Verification items for the finished model (mm, model axes). Coordinates: 2 decimals unless noted, no trailing zeros. Order: outer loops, then holes, each group sorted by start corner. A loop starts at its lowest first (then second) coordinate and runs counter-clockwise, first axis right, second up. Notation, with made-up numbers: M 78.25,62 L 90.25,62 A27 ccw 90.25,80 Z; hole C -6.75,84.25 d1. An arc over 180 degrees is marked long. Return JSON: item names as keys, results as strings. Group by question number.
Q1. Thickness scan on probe 1 along Y at (x, z) = (126.16, 2.05); probe 2 along Y at (x, z) = (33, 0.2); probe 3 along Y at (x, z) = (14, 2.6). Record the ranges inside material, lowest first.
Q2. Section check A-A, the plane z = 1.95. Count the separate pieces of the cut face and the enclosed holes in it, then the cut area to 3 significant figures.
Q3. Go/stop test with flat-tipped pins: pin 1 Ø0.6 at (y, z) = (190, 2) entering from -X; pin 2 Ø1 at (x, z) = (42.5, 1.5) entering from +Y. Record where each tip stops, or that it passes through.
Q4. Mould release check, pull along X, two halves, no side actions. Record for faces 1 (the face through (120.064, 179.912, 1.521)), 2 (the face through (91.605, 168.618, 1.479)), 3 (the face through (93, 63, 3)): pulls with the +X half, pulls with the -X half, needs draft (parallel to the pull), parting line crosses it, or undercut.
Q5. Section check C-C, the plane x = 56.5. Enter the section's corners in (y, z), then the cut area to 3 significant figures.
Q6. Section check B-B, the plane y = -30. Enter the section's corners in (x, z), then the cut area to 3 significant figures.
Autodesk Inventor part; units mm, degrees
ref_plane "YZ Plane" through (0, 0, 0) normal (1, 0, 0) x (0, 1, 0)
ref_plane "XZ Plane" through (0, 0, 0) normal (0, 1, 0) x (-1, 0, 0)
ref_plane "XY Plane" through (0, 0, 0) normal (0, 0, 1) x (1, 0, 0)
sketch "スケッチ1" plane through (0, 0, 0) normal (0, 0, 1) x (1, 0, 0)
  line L0 (0, 0) -> (130.16, 0)
  line L1 (130.16, 0) -> (130.16, 159.597)
  line L2 (130.16, 159.597) -> (0, 159.597)
  line L3 (0, 159.597) -> (0, 0)
  dimension "d0" = 130.16
  dimension "d1" = 159.597
extrude "押し出し1" add sketch "スケッチ1" along normal blind 3
sketch "スケッチ2" plane through (0, 0, 3) normal (0, 0, 1) x (1, 0, 0)
  line L0 (126.16, 3.92) -> (126.16, 113.08) construction
  circle A0 centre (126.16, 3.92) radius 1.6
  circle A1 centre (126.16, 113.08) radius 1.6
  line L1 (130.16, 0) -> (130.16, 159.597)
  line L2 (0, 0) -> (130.16, 0)
  circle A2 centre (121.531, 154.597) radius 1.6
  line L3 (130.16, 159.597) -> (0, 159.597)
  line L4 (121.531, 154.597) -> (121.531, 139.097) construction
  circle A3 centre (121.531, 139.097) radius 1.6
  line L5 (18.398, 154.597) -> (33.898, 154.597) construction
  line L6 (0, 159.597) -> (0, 0) construction
  circle A4 centre (18.398, 154.597) radius 1.6
  circle A5 centre (33.898, 154.597) radius 1.6
  dimension "d4" = 3.2
  dimension "d5" = 4
  dimension "d6" = 3.92
  dimension "d7" = 109.16
  dimension "d10" = 5
  dimension "d11" = 8.629
  dimension "d12" = 15.5
  dimension "d13" = 18.398
  dimension "d14" = 5
  dimension "d15" = 15.5
extrude "押し出し2" cut sketch "スケッチ2" against normal blind 3
sketch "スケッチ9" plane through (0, 0, 3) normal (0, 0, 1) x (1, 0, 0)
  line L0 (130.16, 159.597) -> (0, 159.597)
  line L1 (100.16, 192.597) -> (130.16, 192.597)
  line L2 (130.16, 192.597) -> (130.16, 159.597)
  line L3 (100.16, 192.597) -> (100.16, 187.597)
  line L4 (130.16, 159.597) -> (0, 159.597)
  line L5 (100.16, 187.597) -> (0, 159.597)
  line L6 (130.16, 0) -> (130.16, -147.403)
  line L7 (130.16, -147.403) -> (100.16, -147.403)
  line L8 (100.16, -147.403) -> (100.16, -142.403)
  line L9 (100.16, -142.403) -> (0, 0)
  line L10 (0, 0) -> (130.16, 0)
  circle A0 centre (120.66, 182.597) radius 2.75
  circle A1 centre (120.66, -137.403) radius 2.75
  line L11 (130.16, 192.097) -> (100.16, 192.097)
  line L12 (130.16, -146.903) -> (100.16, -146.903)
  dimension "d50" = 33
  dimension "d51" = 30
  dimension "d52" = 5
  dimension "d53" = 340
  dimension "d54" = 10
  dimension "d55" = 9.5
  dimension "d56" = 0.5
  dimension "d57" = 5.5
  dimension "d58" = 9.5
  dimension "d59" = 10
  dimension "d60" = 0.5
extrude "押し出し8" add sketch "スケッチ9" against normal blind 3 contours L0 L5 L3 L11 L2 | L6 L12 L8 L9 L10
sketch "スケッチ10" plane through (0, 0, 3) normal (0, 0, 1) x (1, 0, 0)
  line L0 (100.16, -146.903) -> (100.16, -142.403)
  line L1 (100.16, -142.403) -> (77.3003, 118.8844)
  line L2 (77.3003, 118.8844) -> (0, 139.597)
  line L3 (0, 159.597) -> (0, 0)
  line L4 (0, 139.597) -> (0, 0)
  line L5 (0, 0) -> (100.16, -142.403)
  line L6 (130.16, -146.903) -> (130.16, 192.097)
  dimension "d63" = 20
  dimension "d64" = 105
  dimension "d65" = 5
extrude "押し出し9" cut sketch "スケッチ10" against normal blind 3
fillet "フィレット2" radius 75 1 edges at (77.3003, 118.8844, 1.5)
sketch "スケッチ12" plane through (0, 0, 3) normal (0, 0, 1) x (1, 0, 0)
  line L0 (100.16, 187.597) -> (100.16, 159.597)
  line L1 (100.16, 159.597) -> (0, 159.597)
  line L2 (0, 159.597) -> (100.16, 187.597)
  line L3 (0, 159.597) -> (0, 139.597)
  point P0 (0, 0)
extrude "押し出し10" cut sketch "スケッチ12" against normal blind 3
fillet "フィレット4" radius 30 1 edges at (100.16, 159.597, 1.5)
fillet "フィレット5" radius 2 5 edges at (100.16, 192.097, 1.5) (0, 159.597, 1.5) (100.16, -146.903, 1.5) (130.16, -146.903, 1.5) (130.16, 192.097, 1.5)
equation "\"d58\" = d55"
equation "\"d59\" = d54"
equation "\"d60\" = d56"
properties part number "small_gpu_05" material "アルミニウム 6061"
Numbers:
{
 "1": {"probe 1": "y = -146.9 to 2.32, 5.52 to 111.48, 114.68 to 192.1", "probe 2": "y = 130.44 to 153.27, 155.92 to 159.6", "probe 3": "y = 135.85 to 159.6"},
 "2": {"separate pieces": "1", "enclosed holes": "8", "area": "17,000 mm2"},
 "3": {"pin 1": "stops at x = 100.16", "pin 2": "stops at y = 159.6"},
 "4": {"face 1": "undercut", "face 2": "pulls with the -X half", "face 3": "needs draft"},
 "5": {"outline": "M 116.52,0 L 159.6,0 L 159.6,3 L 116.52,3 Z", "area": "129 mm2"},
 "6": {"outline": "M 90.33,0 L 130.16,0 L 130.16,3 L 90.33,3 Z", "area": "120 mm2"}
}
